```python
from build123d import *

# Parameters (mm, degrees)
SKICA1_W                 = 25
SKICA1_H                 = 120
P_IDAT_VYSUNUT_M1_DEPTH  = 5
SKICA2_W                 = 25
SKICA2_H                 = 15
P_IDAT_VYSUNUT_M2_DEPTH  = 10
ZAOBLIT5_R               = 5
ZAOBLIT6_R               = 5
ODEBRAT_VYSUNUT_M2_DEPTH = 20
ZAOBLIT7_R               = 10
SKICA4_W                 = 3
SKICA4_H                 = 7
ODEBRAT_VYSUNUT_M3_DEPTH = 4
ODEBRAT_VYSUNUT_M4_DEPTH = 2
ODEBRAT_START            = -3
SKICA7_R                 = 0.5
ODEBRAT_VYSUNUT_M5_DEPTH = 2.8
SKICA8_R                 = 3.75
ODEBRAT_VYSUNUT_M6_DEPTH = 123.837290755
SKICA9_W                 = 7.5
SKICA9_H                 = 8
ODEBRAT_VYSUNUT_M7_DEPTH = 123.983738762


with BuildPart() as part:
    # Skica1 → Přidat vysunutím1 (new body)
    with BuildSketch(Plane.XY):
        with Locations((12.5, 60)):
            Rectangle(SKICA1_W, SKICA1_H)
    extrude(amount=P_IDAT_VYSUNUT_M1_DEPTH)

    # Skica2 → Přidat vysunutím2 (add)
    with BuildSketch(Plane(origin=(0, 0, 0), x_dir=(-1, 0, 0), z_dir=(0, 0, -1))):
        with Locations((-12.5, 112.5)):
            Rectangle(SKICA2_W, SKICA2_H)
    extrude(amount=-P_IDAT_VYSUNUT_M2_DEPTH)

    # Zaoblit5
    zaoblit5_edges = [part.edges().sort_by_distance(p)[0] for p in [
        (25, 0, 2.5),
    ]]
    fillet(zaoblit5_edges, radius=ZAOBLIT5_R)

    # Zaoblit6
    zaoblit6_edges = [part.edges().sort_by_distance(p)[0] for p in [
        (0, 0, 2.5),
    ]]
    fillet(zaoblit6_edges, radius=ZAOBLIT6_R)

    # Skica3 → Odebrat vysunutím2 (cut)
    with BuildSketch(Plane.XY.offset(10)):
        with BuildLine():
            Line((1.5, 118.04), (23.5, 118.04))
            ThreePointArc((23.5, 118.04), (24.1, 118.64), (23.5, 119.24))
            ThreePointArc((23.5, 119.24), (23.12, 119.62), (23.5, 120))
            Line((23.5, 120), (1.5, 120))
            ThreePointArc((1.5, 120), (1.88, 119.62), (1.5, 119.24))
            ThreePointArc((1.5, 119.24), (0.9, 118.64), (1.5, 118.04))
        make_face()
    extrude(amount=-ODEBRAT_VYSUNUT_M2_DEPTH, mode=Mode.SUBTRACT)

    # Zaoblit7
    # the kernel refuses this fillet: 10 mm, written as the material it takes off along each edge
    with BuildSketch(Plane(origin=(-21.650635095, 105, 10), x_dir=(0, 0, -1), z_dir=(1, 0, 0))) as zaoblit7_piece_1:
        with BuildLine():
            CenterArc((10, 8.660254038), ZAOBLIT7_R, 180, 60)
            Line((0, 8.660254038), (-0.2, 8.660254038))
            Line((-0.2, 8.660254038), (-0.2, 0))
            Line((-0.2, 0), (0, -0.2))
            ThreePointArc((0, -0.2), (2.5, -0.2), (4.9, -0.173205081))
            Line((4.9, -0.173205081), (5, 0))
        make_face()
    extrude(amount=68.301270189, mode=Mode.SUBTRACT)

    # Zaoblit8
    # the kernel refuses this chamfer: 2 mm, written as the material it adds along each edge
    with BuildSketch(Plane(origin=(25, 105, 5), x_dir=(0, -0.9995029762160257, -0.031524602064212835), z_dir=(-1, 0, 0))) as zaoblit8_piece_1:
        with BuildLine():
            Line((1.15829653, 0), (-0.636224816, 0.850214013))
            Line((-0.636224816, 0.850214013), (-0.667962409, 0.825868064))
            ThreePointArc((-0.667962409, 0.825868064), (-0.324476703, 0.420675743), (-0.033993307, -0.021082104))
            Line((-0.033993307, -0.021082104), (0.001260984, -0.039980119))
            ThreePointArc((0.001260984, -0.039980119), (0.579833691, -0.021731775), (1.159557514, -0.039980119))
            Line((1.159557514, -0.039980119), (1.15829653, 0))
        make_face()
    extrude(amount=25)

    # Skica4 → Odebrat vysunutím3 (cut)
    with BuildSketch(Plane(origin=(0, 118.04, 0), x_dir=(1, 0, 0), z_dir=(0, 1, 0))):
        with Locations((9.62, -3.5)):
            Rectangle(SKICA4_W, SKICA4_H)
    extrude(amount=-ODEBRAT_VYSUNUT_M3_DEPTH, mode=Mode.SUBTRACT)

    # Skica5 → Odebrat vysunutím4 (cut)
    with BuildSketch(Plane.XY):
        Polygon((11, 43), (9.272727273, 24), (15.727272727, 24), (14, 43), align=None)
        with BuildLine():
            Line((5.5, 24), (5.5, 20))
            ThreePointArc((5.5, 20), (3.5, 22), (5.5, 24))
        make_face()
        Polygon((9.09375, 20), (9, 21), (9.272727273, 24), (5.5, 24), (5.5, 20), align=None)
        Polygon((9.272727273, 24), (9, 21), (16, 21), (15.727272727, 24), align=None)
        Polygon((16, 21), (9, 21), (9.09375, 20), (15.90625, 20), align=None)
        Polygon((15.727272727, 24), (16, 21), (15.90625, 20), (19.5, 20), (19.5, 24), align=None)
        with BuildLine():
            ThreePointArc((19.5, 24), (21.5, 22), (19.5, 20))
            Line((19.5, 20), (19.5, 24))
        make_face()
        Polygon((15.90625, 20), (9.09375, 20), (10.5, 5), (14.5, 5), align=None)
    extrude(amount=ODEBRAT_VYSUNUT_M4_DEPTH, mode=Mode.SUBTRACT)

    # Skica7 → Odebrat vysunutím5 (cut)
    with BuildSketch(Plane(origin=(0, 0, 2), x_dir=(-1, 0, 0), z_dir=(0, 0, -1)).offset(ODEBRAT_START)):
        with Locations(Location((-12.5, 36.2, 0), (0, 0, 180))):
            Circle(SKICA7_R)
        with Locations(Location((-12.5, 9.7, 0), (0, 0, 180))):
            Circle(SKICA7_R)
    extrude(amount=ODEBRAT_VYSUNUT_M5_DEPTH, mode=Mode.SUBTRACT)

    # Skica8 → Odebrat vysunutím6 (cut, through all)
    with BuildSketch(Plane(origin=(0, 0, 2), x_dir=(-1, 0, 0), z_dir=(0, 0, -1))):
        with Locations((-12.5, 22)):
            Circle(SKICA8_R)
    extrude(amount=-ODEBRAT_VYSUNUT_M6_DEPTH, mode=Mode.SUBTRACT)

    # Skica9 → Odebrat vysunutím7 (cut, through all)
    with BuildSketch(Plane(origin=(0, 0, 0), x_dir=(-1, 0, 0), z_dir=(0, 0, -1))):
        with Locations((-19.65625, 16)):
            Rectangle(SKICA9_W, SKICA9_H)
    extrude(amount=-ODEBRAT_VYSUNUT_M7_DEPTH, mode=Mode.SUBTRACT)


solid = part.part
```
Geometry: final body of the model. Coordinates: model frame, mm. A direction names the side the tool comes from. Coordinates: 2 decimals unless noted, no trailing zeros. Order: outer loops, then holes, each group sorted by start corner. A loop starts at its lowest first (then second) coordinate and runs counter-clockwise, first axis right, second up. Notation, with made-up numbers: (87.5, 69.25) - (126.5, 69.25) arc R9 cw to (126.5, 83.25) - close; hole circle Ø3 at (35, 22.25). An arc over 180 degrees is marked (long way). Return JSON: item names as keys, results as strings. Group by question number.
1. Material intervals for line 1 along Y through (x, z) = (12.5, 3.9); line 2 along X through (y, z) = (9.7, 3.6); line 3 along Z through (x, y) = (8.75, 48.5), sorted ascending. Write a range as [from, to].
2. Pin query (flat end, axial travel): pin 1 (2.5 mm diameter, centred on x = 9.5, y = 116.5, fed in from -Z); pin 2 (1 mm diameter, centred on x = 19, y = 53.5, fed in from +Z); pin 3 (1.2 mm diameter, centred on y = 115.5, z = 2.5, fed in from -X); pin 4 (4.5 mm diameter, centred on x = 12.5, y = 22, fed in from +Z). Return the tip coordinate at first contact, or that it passes through.
3. Pull-direction query (X, two-part tool) for faces 4 (the face through (0, 62, 3)), 5 (the face through (12, 53, 5)), 6 (the face through (15.193, 12.395, 0.986)); classes: pulls with the +X half, pulls with the -X half, needs draft (parallel to the pull), parting line crosses it, or undercut.
4. Cut plane C-C (y = 16.5). Output: boundary loops of the cut face in (x, z).
5. Cut plane D-D (y = 72.5). Output: boundary loops of the cut face in (x, z).
6. Set-up query: faces 1 (the face through (3.5, 22, 1)), 2 (the face through (13, 116, 10)), 3 (the face through (15.906, 16, 2)). Return all of +Z, -Z, +X, -X, +Y, -Y with unobstructed straight access to the full face (end or side cutting, diameter ignored); none if empty.
7. Cut plane A-A (x = 18.5). Output: boundary loops of the cut face in (y, z), plus the area to 3 significant figures.
Resolved:
{
 "1": {"line 1": "y = [0, 9.2], [10.2, 18.25], [25.75, 35.7], [36.7, 118.04]", "line 2": "x = [0, 12], [13, 25]", "line 3": "z = [0, 5]"},
 "2": {"pin 1": "stops at z = 7", "pin 2": "stops at z = 5", "pin 3": "stops at x = 0", "pin 4": "passes through"},
 "3": {"face 4": "pulls with the -X half", "face 5": "needs draft", "face 6": "undercut"},
 "4": {"outline": "(0, 0) - (9.42, 0) - (9.42, 2) - (15.58, 2) - (15.58, 0) - (15.91, 0) - (15.91, 5) - (0, 5) - close; (23.41, 0) - (25, 0) - (25, 5) - (23.41, 5) - close"},
 "5": {"outline": "(0, 0) - (25, 0) - (25, 5) - (0, 5) - close"},
 "6": {"face 1": "-Z", "face 2": "+Z, +X, -X, +Y, -Y", "face 3": "+Z, -Z"},
 "7": {"outline": "(0, 0) - (12, 0) - (12, 5) - (0, 5) - close; (20, 2) - (24, 2) - (24, 0) - (118.04, 0) - (118.04, 10) - (113.66, 10) arc R10 ccw to (105.54, 5.83) - (103.91, 5) - (20, 5) - close", "area": "595 mm²"}
}
